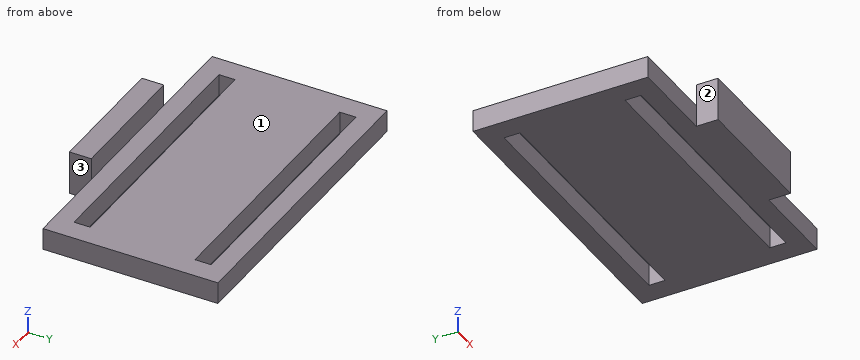
```python
from build123d import *

# Parameters (mm, degrees)
F0_W     = 88.9
F0_H     = 50.8
F0_W_2   = 76.2
F0_H_2   = 4.70328
F1_DEPTH = 6.35
F2_W     = 38.1
F2_H     = 6.35
F3_DEPTH = 6.35
F4_W     = 38.1
F4_H     = 6.35
F5_DEPTH = 6.35


with BuildPart() as f1:
    # F0 (on Top) → F1 (new body)
    with BuildSketch(Plane.XY):
        Rectangle(F0_W, F0_H)
        with Locations((0, -17.556932)):
            Rectangle(F0_W_2, F0_H_2, mode=Mode.SUBTRACT)
        with Locations((0, 17.556932)):
            Rectangle(F0_W_2, F0_H_2, mode=Mode.SUBTRACT)
    extrude(amount=F1_DEPTH)

    # F2 (on face) → F3 (join)
    with BuildSketch(Plane.XZ.offset(25.4)):
        with Locations((0, 3.175)):
            Rectangle(F2_W, F2_H)
    extrude(amount=F3_DEPTH)

    # F4 (on face) → F5 (join)
    with BuildSketch(Plane.XY.offset(6.35)):
        with Locations((0, -28.575)):
            Rectangle(F4_W, F4_H)
    extrude(amount=F5_DEPTH)


solid = f1.part
```
Could you check a few things on this model? Use its own coordinates, in mm. Face numbers are marked on the shaded views. A direction names the side the tool comes from. Round coordinates to 2 decimals unless told otherwise and drop trailing zeros. Loops run counter-clockwise (first coordinate to the right, second up) from the corner with the lowest first, then second, coordinate; pieces in that order, holes last. Notation, with made-up numbers: (-38.5, 59.5) - (-21.5, 59.5) arc R8 ccw to (-21.5, 71.5) - close; hole circle Ø10 at (63, -28). An arc over 180 degrees is marked (long way). Answer as CSV lines item,"result".
1. I want a section at D-D on y = 8.5. List the corners of the cut face in (x, z) for me.
Filled in:
outline,"(-44.45, 0) - (44.45, 0) - (44.45, 6.35) - (-44.45, 6.35) - close"
2. Please list where these lines run through material, in increasing order: line 1 along Y through (x, z) = (9, 5); line 2 along Y through (x, z) = (19.5, 3.5); line 3 along X through (y, z) = (-19, 2.25). Write a range as [from, to].
Filled in:
line 1,"y = [-31.75, -19.91], [-15.21, 15.21], [19.91, 25.4]"
line 2,"y = [-25.4, -19.91], [-15.21, 15.21], [19.91, 25.4]"
line 3,"x = [-44.45, -38.1], [38.1, 44.45]"
3. On a 3-axis mill with a long thin cutter (end or side, diameter ignored), from which of +Z, -Z, +X, -X, +Y, -Y can I reach the whole of each face in a straight line? I mean the marked faces 1, 2 and 3. Say none if no direction works.
Filled in:
face 1,"+Z, +X, -X, +Y"
face 2,"+Z, -Z, -X, -Y"
face 3,"+Z, -Z, +X, -Y"
4. For pin 1 Ø2 at (x, y) = (20, 3.5) entering from +Z; pin 2 Ø1.9 at (y, z) = (-27, 4) entering from +X; pin 3 Ø6 at (x, z) = (29, 11) entering from +Y; pin 4 Ø1.9 at (x, z) = (31.5, 2) entering from -Y, each with a flat end and sliding along its axis, tell me the tip position at first contact or that it passes through.
Filled in:
pin 1,"stops at z = 6.35"
pin 2,"stops at x = 19.05"
pin 3,"passes through"
pin 4,"stops at y = -25.4"
5. I want a section at A-A on x = -37. List the corners of the cut face in (y, z) for me.
Filled in:
outline,"(-25.4, 0) - (-19.91, 0) - (-19.91, 6.35) - (-25.4, 6.35) - close; (-15.21, 0) - (15.21, 0) - (15.21, 6.35) - (-15.21, 6.35) - close; (19.91, 0) - (25.4, 0) - (25.4, 6.35) - (19.91, 6.35) - close"
6. I want a section at C-C on x = -6. List the corners of the cut face in (y, z) for me.
Filled in:
outline,"(-31.75, 0) - (-19.91, 0) - (-19.91, 6.35) - (-25.4, 6.35) - (-25.4, 12.7) - (-31.75, 12.7) - close; (-15.21, 0) - (15.21, 0) - (15.21, 6.35) - (-15.21, 6.35) - close; (19.91, 0) - (25.4, 0) - (25.4, 6.35) - (19.91, 6.35) - close"
7. I want a section at B-B on z = 4.5. List the corners of the cut face in (x, y) for me, then the cut area to 3 significant figures.
Filled in:
outline,"(-44.45, -25.4) - (-19.05, -25.4) - (-19.05, -31.75) - (19.05, -31.75) - (19.05, -25.4) - (44.45, -25.4) - (44.45, 25.4) - (-44.45, 25.4) - close; hole (-38.1, -19.91) - (38.1, -19.91) - (38.1, -15.21) - (-38.1, -15.21) - close; hole (-38.1, 15.21) - (38.1, 15.21) - (38.1, 19.91) - (-38.1, 19.91) - close"
area,"4,040 mm^2"
